Check sheet for the modelled part. Datum: model origin and axes. Units: mm. A direction names the side the tool comes from. Give positions to 0.01 mm unless a question says otherwise; leave off trailing zeros. Loops run counter-clockwise (first coordinate to the right, second up) from the corner with the lowest first, then second, coordinate; pieces in that order, holes last. Notation, with made-up numbers: (6, -24) - (30, -24) arc R35 ccw to (30, 13) - close; hole circle Ø11 at (-20.5, -33). An arc over 180 degrees is marked (long way). Use one line per item in the form item = value.
from build123d import *

# Parameters (mm, degrees)
F1_DEPTH = 41
F2_R     = 2.2
F3_R     = 0.7
F4_R     = 1
F5_DEPTH = 33.501
F6_R     = 1
F7_R     = 5.25
F7_R_2   = 1
F8_DEPTH = 1.5


with BuildPart() as f1:
    # F0 (on Top) → F1 (new body)
    with BuildSketch(Plane.XY):
        Polygon((-16.75, -5.75), (16.75, -5.75), (16.75, 5.75), (15.25, 5.75), (15.25, -4.25), (-15.25, -4.25), (-15.25, 5.75), (-16.75, 5.75), align=None)
    extrude(amount=F1_DEPTH)

    # F2
    f2_edges = [f1.edges().sort_by_distance(p)[0] for p in [
        (16.75, -5.75, 20.5),
        (-16.75, -5.75, 20.5),
    ]]
    fillet(f2_edges, radius=F2_R)

    # F3
    f3_edges = [f1.edges().sort_by_distance(p)[0] for p in [
        (-15.25, -4.25, 20.5),
        (15.25, -4.25, 20.5),
    ]]
    fillet(f3_edges, radius=F3_R)

    # F4 (on face) → F5 (cut, through all)
    with BuildSketch(Plane.YZ.offset(16.75)):
        with Locations((2.75, 38.5)):
            Circle(F4_R)
        with Locations((2.75, 2.5)):
            Circle(F4_R)
    extrude(amount=-F5_DEPTH, mode=Mode.SUBTRACT)

    # F6
    f6_edges = [f1.edges().sort_by_distance(p)[0] for p in [
        (-16, 5.75, 41),
        (16, 5.75, 41),
        (-16, 5.75, 0),
        (16, 5.75, 0),
    ]]
    fillet(f6_edges, radius=F6_R)

    # F7 (on face) → F8 (cut, through all)
    with BuildSketch(Plane(origin=(0, -4.25, 0), x_dir=(-1, 0, 0), z_dir=(0, 1, 0))):
        with Locations((0, 20.5)):
            Circle(F7_R)
        with Locations((0, 27.5)):
            Circle(F7_R_2)
        with Locations((-4.949747, 25.449747)):
            Circle(F7_R_2)
        with Locations((-7, 20.5)):
            Circle(F7_R_2)
        with Locations((-4.949747, 15.550253)):
            Circle(F7_R_2)
        with Locations((0, 13.5)):
            Circle(F7_R_2)
        with Locations((4.949747, 15.550253)):
            Circle(F7_R_2)
        with Locations((7, 20.5)):
            Circle(F7_R_2)
        with Locations((4.949747, 25.449747)):
            Circle(F7_R_2)
    extrude(amount=-F8_DEPTH, mode=Mode.SUBTRACT)


solid = f1.part
Item 1: Section check B-B on x = 0. Record the boundary of the cut face in (y, z), then the cut area to 4 significant figures.
Answer block:
outline = (-5.75, 0) - (-4.25, 0) - (-4.25, 12.5) - (-5.75, 12.5) - close; (-5.75, 14.5) - (-4.25, 14.5) - (-4.25, 15.25) - (-5.75, 15.25) - close; (-5.75, 25.75) - (-4.25, 25.75) - (-4.25, 26.5) - (-5.75, 26.5) - close; (-5.75, 28.5) - (-4.25, 28.5) - (-4.25, 41) - (-5.75, 41) - close
area = 39.75 mm2
Item 2: Section check A-A on y = 0.75. Record the boundary of the cut face in (x, z).
Answer block:
outline = (-16.75, 0) - (-15.25, 0) - (-15.25, 41) - (-16.75, 41) - close; (15.25, 0) - (16.75, 0) - (16.75, 41) - (15.25, 41) - close
Item 3: Access from +Z, -Z, +X, -X, +Y, -Y to the whole of each face (thin tool, end or side, straight path). Record for faces 1 (the face through (-6.783, -4.99, 19.524)), 2 (the face through (15.25, 1, 20)).
Answer block:
face_1 = +Y, -Y
face_2 = +Z, -Z, +Y
Item 4: Section check D-D on x = -7. Record the boundary of the cut face in (y, z), then the cut area to 3 significant figures.
Answer block:
outline = (-5.75, 0) - (-4.25, 0) - (-4.25, 19.5) - (-5.75, 19.5) - close; (-5.75, 21.5) - (-4.25, 21.5) - (-4.25, 41) - (-5.75, 41) - close
area = 58.5 mm2
Item 5: Thickness scan on L1, parallel to Z at x = 16.25, y = 2.75; L2, parallel to X at y = -0.75, z = 7; L3, parallel to Y at x = 7, z = 28. Record the ranges inside material, lowest first.
Answer block:
L1 = 0 to 1.5, 3.5 to 37.5, 39.5 to 41
L2 = -16.75 to -15.25, 15.25 to 16.75
L3 = -5.75 to -4.25
Item 6: Mould release check, pull along Y, two halves, no side actions. Record for faces 3 (the face through (16.09, -5.12, 20.79)), 4 (the face through (16.01, 2.62, 39.49)), 5 (the face through (15.99, 5.449, 0.285)), 6 (the face through (-16.75, 1, 20)): released by +Y, released by -Y, zero draft, split by the parting line, or undercut.
Answer block:
face_3 = released by -Y
face_4 = undercut
face_5 = released by +Y
face_6 = zero draft
Item 7: Gauge pin test, flat ends, axial feed: P1, Ø1.2, axis at x = -4.95, z = 25.45, coming from the +Y side; P2, Ø2.5, axis at x = 0, z = 13.5, coming from the +Y side. Record the tip position at first contact, or that the pin passes through.
Answer block:
P1 = through
P2 = -4.25
Item 8: Section check C-C on z = 13.5. Record the boundary of the cut face in (x, y).
Answer block:
outline = (-16.75, -3.55) arc R2.2 ccw to (-14.55, -5.75) - (-1, -5.75) - (-1, -4.25) - (-14.55, -4.25) arc R0.7 cw to (-15.25, -3.55) - (-15.25, 5.75) - (-16.75, 5.75) - close; (1, -5.75) - (14.55, -5.75) arc R2.2 ccw to (16.75, -3.55) - (16.75, 5.75) - (15.25, 5.75) - (15.25, -3.55) arc R0.7 cw to (14.55, -4.25) - (1, -4.25) - close
